The listing builds one solid part. Answer for the finished solid, in the listing's coordinates (mm). A direction names the side the tool comes from. Coordinates: 2 decimals unless noted, no trailing zeros. Loops run counter-clockwise (first coordinate to the right, second up) from the corner with the lowest first, then second, coordinate; pieces in that order, holes last. Notation, with made-up numbers: (71.5, -16.5) - (87.5, -16.5) arc R17 ccw to (87.5, 9.5) - close; hole circle Ø1 at (72.25, 10.5). An arc over 180 degrees is marked (long way). One line per question, with ' | ' between items.
from build123d import *

# Parameters (mm, degrees)
SKETCH1_W           = 85.8
SKETCH1_H           = 92.5
BOSS_EXTRUDE1_DEPTH = 14.859
SKETCH2_W           = 85.8
SKETCH2_H           = 92.5
SKETCH2_R           = 1
BOSS_EXTRUDE2_DEPTH = 3.175
SKETCH4_W           = 85.8
SKETCH4_H           = 92.5
SKETCH4_W_2         = 75.8
SKETCH4_H_2         = 82.5
BOSS_EXTRUDE3_DEPTH = 4.5
CUT_EXTRUDE1_DEPTH  = 121.663419813
SKETCH5_W           = 14
SKETCH5_H           = 8
CUT_EXTRUDE2_DEPTH  = 121.663419813
SKETCH6_W           = 10
SKETCH6_H           = 6
CUT_EXTRUDE3_DEPTH  = 121.663419813
BOSS_EXTRUDE4_START = 1.9
SKETCH7_R           = 3.54
SKETCH7_R_2         = 1
BOSS_EXTRUDE4_DEPTH = 1.9
FILLET1_R           = 2.5
FILLET2_R           = 2.5
FILLET3_R           = 2.5
FILLET4_R           = 2.5
FILLET5_R           = 2.5


with BuildPart() as part:
    # Sketch1 → Boss-Extrude1 (new body)
    with BuildSketch(Plane(origin=(0, 0, 0), x_dir=(1, 0, 0), z_dir=(0, 1, 0))):
        with Locations((37.9, 41.25)):
            Rectangle(SKETCH1_W, SKETCH1_H)
        Polygon((5, 4), (5, 10), (0, 10), (0, 82.5), (70.8, 82.5), (70.8, 79), (75.8, 79), (75.8, 4), (59.9, 4), (59.9, 0), (52.9, 0), (52.9, 4), (41.4, 4), (41.4, 0), (34.4, 0), (34.4, 4), (22.9, 4), (22.9, 0), (15.9, 0), (15.9, 4), align=None, mode=Mode.SUBTRACT)
    extrude(amount=BOSS_EXTRUDE1_DEPTH)

    # Sketch2 → Boss-Extrude2 (add)
    with BuildSketch(Plane(origin=(0, 0, 0), x_dir=(1, 0, 0), z_dir=(0, 1, 0))):
        with Locations((37.9, 41.25)):
            Rectangle(SKETCH2_W, SKETCH2_H)
        with Locations(Location((3.5, 13.5, 0), (0, 0, 270))):
            Circle(SKETCH2_R, mode=Mode.SUBTRACT)
        with Locations(Location((19.4, 3.5, 0), (0, 0, 270))):
            Circle(SKETCH2_R, mode=Mode.SUBTRACT)
        with Locations(Location((37.9, 3.5, 0), (0, 0, 270))):
            Circle(SKETCH2_R, mode=Mode.SUBTRACT)
        with Locations(Location((56.4, 3.5, 0), (0, 0, 270))):
            Circle(SKETCH2_R, mode=Mode.SUBTRACT)
        with Locations(Location((30.3, 56.1, 0), (0, 0, 270))):
            Circle(SKETCH2_R, mode=Mode.SUBTRACT)
        with Locations(Location((71.8, 75.5, 0), (0, 0, 270))):
            Circle(SKETCH2_R, mode=Mode.SUBTRACT)
    extrude(amount=-BOSS_EXTRUDE2_DEPTH)

    # Sketch4 → Boss-Extrude3 (add)
    with BuildSketch(Plane(origin=(0, 14.859, 0), x_dir=(1, 0, 0), z_dir=(0, 1, 0))):
        with Locations((37.9, 41.25)):
            Rectangle(SKETCH4_W, SKETCH4_H)
        with Locations((37.9, 41.25)):
            Rectangle(SKETCH4_W_2, SKETCH4_H_2, mode=Mode.SUBTRACT)
    extrude(amount=BOSS_EXTRUDE3_DEPTH)

    # Sketch3 → Cut-Extrude1 (cut, through all)
    with BuildSketch(Plane(origin=(0, 0, 0), x_dir=(0, 0, -1), z_dir=(1, 0, 0))):
        with BuildLine():
            Line((60.6, 14.859), (60.6, 19.359))
            Line((60.6, 19.359), (51.6, 19.359))
            Line((51.6, 19.359), (51.6, 14.859))
            ThreePointArc((51.6, 14.859), (56.1, 10.359), (60.6, 14.859))
        make_face()
    extrude(amount=-CUT_EXTRUDE1_DEPTH, mode=Mode.SUBTRACT)

    # Sketch5 → Cut-Extrude2 (cut, through all)
    with BuildSketch(Plane.XY):
        with Locations((10.15, 20)):
            Rectangle(SKETCH5_W, SKETCH5_H)
        with Locations((28.65, 20)):
            Rectangle(SKETCH5_W, SKETCH5_H)
        with Locations((47.15, 20)):
            Rectangle(SKETCH5_W, SKETCH5_H)
        with Locations((65.65, 20)):
            Rectangle(SKETCH5_W, SKETCH5_H)
    extrude(amount=CUT_EXTRUDE2_DEPTH, mode=Mode.SUBTRACT)

    # Sketch6 → Cut-Extrude3 (cut, through all)
    with BuildSketch(Plane.XY):
        with Locations((59, 19.383)):
            Rectangle(SKETCH6_W, SKETCH6_H)
    extrude(amount=-CUT_EXTRUDE3_DEPTH, mode=Mode.SUBTRACT)

    # Sketch7 → Boss-Extrude4 (add)
    # profile 1 of 6: a face of its own
    with BuildSketch(Plane(origin=(0, 0, 0), x_dir=(1, 0, 0), z_dir=(0, 1, 0)).offset(BOSS_EXTRUDE4_START)):
        with Locations(Location((30.3, 56.1, 0), (0, 0, 90))):
            Circle(SKETCH7_R)
        with Locations(Location((30.3, 56.1, 0), (0, 0, 270))):
            Circle(SKETCH7_R_2, mode=Mode.SUBTRACT)
    # profile 2 of 6: a face of its own
    with BuildSketch(Plane(origin=(0, 0, 0), x_dir=(1, 0, 0), z_dir=(0, 1, 0)).offset(BOSS_EXTRUDE4_START)):
        with BuildLine():
            Line((0, 13.5), (0, 10))
            Line((0, 10), (3.5, 10))
            ThreePointArc((3.5, 10), (5.974873734, 15.974873734), (0, 13.5))
        make_face()
        with Locations(Location((3.5, 13.5, 0), (0, 0, 270))):
            Circle(SKETCH7_R_2, mode=Mode.SUBTRACT)
    # profile 3 of 6: a face of its own
    with BuildSketch(Plane(origin=(0, 0, 0), x_dir=(1, 0, 0), z_dir=(0, 1, 0)).offset(BOSS_EXTRUDE4_START)):
        with BuildLine():
            Line((15.9, 3.5), (15.9, 0))
            Line((15.9, 0), (22.9, 0))
            Line((22.9, 0), (22.9, 3.5))
            ThreePointArc((22.9, 3.5), (19.4, 7), (15.9, 3.5))
        make_face()
        with Locations(Location((19.4, 3.5, 0), (0, 0, 270))):
            Circle(SKETCH7_R_2, mode=Mode.SUBTRACT)
    # profile 4 of 6: a face of its own
    with BuildSketch(Plane(origin=(0, 0, 0), x_dir=(1, 0, 0), z_dir=(0, 1, 0)).offset(BOSS_EXTRUDE4_START)):
        with BuildLine():
            Line((34.4, 3.5), (34.4, 0))
            Line((34.4, 0), (41.4, 0))
            Line((41.4, 0), (41.4, 3.5))
            ThreePointArc((41.4, 3.5), (37.9, 7), (34.4, 3.5))
        make_face()
        with Locations(Location((37.9, 3.5, 0), (0, 0, 270))):
            Circle(SKETCH7_R_2, mode=Mode.SUBTRACT)
    # profile 5 of 6: a face of its own
    with BuildSketch(Plane(origin=(0, 0, 0), x_dir=(1, 0, 0), z_dir=(0, 1, 0)).offset(BOSS_EXTRUDE4_START)):
        with BuildLine():
            Line((52.9, 3.5), (52.9, 0))
            Line((52.9, 0), (59.9, 0))
            Line((59.9, 0), (59.9, 3.5))
            ThreePointArc((59.9, 3.5), (56.4, 7), (52.9, 3.5))
        make_face()
        with Locations(Location((56.4, 3.5, 0), (0, 0, 270))):
            Circle(SKETCH7_R_2, mode=Mode.SUBTRACT)
    # profile 6 of 6: a face of its own
    with BuildSketch(Plane(origin=(0, 0, 0), x_dir=(1, 0, 0), z_dir=(0, 1, 0)).offset(BOSS_EXTRUDE4_START)):
        with BuildLine():
            Line((75.8, 79), (69.863508327, 79))
            ThreePointArc((69.863508327, 79), (69.768493994, 72.054280431), (75.8, 75.5))
            Line((75.8, 75.5), (75.8, 79))
        make_face()
        with Locations(Location((71.8, 75.5, 0), (0, 0, 270))):
            Circle(SKETCH7_R_2, mode=Mode.SUBTRACT)
    extrude(amount=-BOSS_EXTRUDE4_DEPTH)

    # Fillet1
    fillet1_edges = [part.edges().sort_by_distance(p)[0] for p in [
        (-5, 8.092, 5),
    ]]
    fillet(fillet1_edges, radius=FILLET1_R)

    # Fillet2
    fillet2_edges = [part.edges().sort_by_distance(p)[0] for p in [
        (80.8, 8.092, 5),
    ]]
    fillet(fillet2_edges, radius=FILLET2_R)

    # Fillet3
    fillet3_edges = [part.edges().sort_by_distance(p)[0] for p in [
        (80.8, 8.092, -87.5),
    ]]
    fillet(fillet3_edges, radius=FILLET3_R)

    # Fillet4
    fillet4_edges = [part.edges().sort_by_distance(p)[0] for p in [
        (-5, 8.092, -87.5),
    ]]
    fillet(fillet4_edges, radius=FILLET4_R)

    # Fillet5
    fillet5_edges = [part.edges().sort_by_distance(p)[0] for p in [
        (37.9, -3.175, 5),
        (-4.267766953, -3.175, 4.267766953),
        (80.8, -3.175, -41.25),
        (80.067766953, -3.175, 4.267766953),
        (37.9, -3.175, -87.5),
        (80.067766953, -3.175, -86.767766953),
        (-5, -3.175, -41.25),
        (-4.267766953, -3.175, -86.767766953),
    ]]
    fillet(fillet5_edges, radius=FILLET5_R)


solid = part.part
Item 1: Find the intervals of material crossed by line 1 (X direction, y = -0.65, z = -3.5); line 2 (X direction, y = 3.75, z = -3.5); line 3 (X direction, y = -0.75, z = -13.5), in increasing order. Write a range as [from, to].
Taken from the geometry:
line 1: x = [-5, 18.4], [20.4, 36.9], [38.9, 55.4], [57.4, 80.8] | line 2: x = [-5, 15.9], [22.9, 34.4], [41.4, 52.9], [59.9, 80.8] | line 3: x = [-5, 2.5], [4.5, 80.8]
Item 2: Find section A-A, the plane y = 4.75. Write down the section's boundary in (x, z).
Taken from the geometry:
outline: (-5, -85) arc R2.5 ccw to (-2.5, -87.5) - (78.3, -87.5) arc R2.5 ccw to (80.8, -85) - (80.8, 2.5) arc R2.5 ccw to (78.3, 5) - (-2.5, 5) arc R2.5 ccw to (-5, 2.5) - close; hole (0, -82.5) - (70.8, -82.5) - (70.8, -79) - (75.8, -79) - (75.8, -4) - (59.9, -4) - (59.9, 0) - (52.9, 0) - (52.9, -4) - (41.4, -4) - (41.4, 0) - (34.4, 0) - (34.4, -4) - (22.9, -4) - (22.9, 0) - (15.9, 0) - (15.9, -4) - (5, -4) - (5, -10) - (0, -10) - close
Item 3: Each of these flat-tipped pins is pushed along its axis until it touches: pin 1 Ø4 at (x, z) = (67.5, 3) entering from +Y; pin 2 Ø12 at (x, z) = (23.5, -74.5) entering from +Y; pin 3 Ø8 at (x, z) = (31, -57.5) entering from +Y. Where does it stop, or does it pass through?
Taken from the geometry:
pin 1: stops at y = 16 | pin 2: stops at y = 0 | pin 3: stops at y = 1.9
Item 4: The mould has two halves that part along Z. Classify faces 1 (the face through (3.15, 18, 2)), 2 (the face through (56.5, 1, -7)), 3 (the face through (37, 9, -87.5)): pulls with the +Z half, pulls with the -Z half, needs draft (parallel to the pull), parting line crosses it, or undercut.
Taken from the geometry:
face 1: needs draft | face 2: undercut | face 3: pulls with the -Z half
Item 5: Find section B-B, the plane z = -65. Write down the section's boundary in (x, y) (3 decimals), plus the area to 3 significant figures.
Taken from the geometry:
outline: (-5, -0.675) arc R2.5 ccw to (-2.5, -3.175) - (78.3, -3.175) arc R2.5 ccw to (80.8, -0.675) - (80.8, 19.359) - (75.8, 19.359) - (75.8, 0) - (0, 0) - (0, 19.359) - (-5, 19.359) - close | area: 463 mm2
Item 6: Find section C-C, the plane x = 14. Write down the section's boundary in (y, z) (3 decimals), plus the area to 3 significant figures.
Taken from the geometry:
outline: (-3.175, -85) arc R2.5 ccw to (-0.675, -87.5) - (19.359, -87.5) - (19.359, -82.5) - (0, -82.5) - (0, -4) - (14.859, -4) - (14.859, 0) - (16, 0) - (16, 5) - (-0.675, 5) arc R2.5 ccw to (-3.175, 2.5) - close | area: 527 mm2
Item 7: Which of the six approach directions +Z, -Z, +X, -X, +Y, -Y give full straight-line access (tool end or side, diameter ignored) to faces 4 (the face through (56, 1.9, -2)), 5 (the face through (59, 16.383, -85)), 6 (the face through (29, 16, 2))?
Taken from the geometry:
face 4: +Y | face 5: -Z, +Y | face 6: +Z, +Y
